```python
from build123d import *

# Parameters (mm, degrees)
SKETCH1_W           = 44.4
SKETCH1_H           = 40
SKETCH1_R           = 2.6
BOSS_EXTRUDE1_DEPTH = 2
SKETCH2_W           = 44.4
SKETCH2_H           = 18.3
BOSS_EXTRUDE2_DEPTH = 2
LPATTERN1_COUNT     = 2
LPATTERN1_PITCH     = 16.3
SKETCH3_R           = 2.6
CUT_EXTRUDE1_DEPTH  = 64.253853638
BOSS_EXTRUDE3_START = -22.2
SKETCH6_W           = 11.69
SKETCH6_H           = 16
BOSS_EXTRUDE3_DEPTH = 44.4
FILLET4_SIZE        = 1
SKETCH11_W          = 10
SKETCH11_H          = 5
CUT_EXTRUDE6_DEPTH  = 14
SKETCH12_W          = 10
SKETCH12_H          = 8.384441544
CUT_EXTRUDE7_DEPTH  = 11
SKETCH7_R           = 2.6
CUT_EXTRUDE2_DEPTH  = 9


with BuildPart() as part:
    # Sketch1 → Boss-Extrude1 (new body)
    with BuildSketch(Plane.XY):
        with Locations((22.2, 20)):
            Rectangle(SKETCH1_W, SKETCH1_H)
        with Locations((8, 8.476902454)):
            Circle(SKETCH1_R, mode=Mode.SUBTRACT)
        with Locations((8, 29.976902454)):
            Circle(SKETCH1_R, mode=Mode.SUBTRACT)
        with Locations((36.4, 29.976902454)):
            Circle(SKETCH1_R, mode=Mode.SUBTRACT)
        with Locations((36.4, 8.476902454)):
            Circle(SKETCH1_R, mode=Mode.SUBTRACT)
    boss_extrude1 = extrude(amount=BOSS_EXTRUDE1_DEPTH)

    # Sketch2 → Boss-Extrude2 (add)
    with BuildSketch(Plane(origin=(0, 40, 0), x_dir=(1, 0, 0), z_dir=(0, 1, 0))):
        with Locations((22.2, 7.15)):
            Rectangle(SKETCH2_W, SKETCH2_H)
    extrude(amount=BOSS_EXTRUDE2_DEPTH)

    # LPattern1: Boss-Extrude1 ×2
    with Locations(*[(0, 0, -i * LPATTERN1_PITCH) for i in range(1, LPATTERN1_COUNT)]):
        add(boss_extrude1)

    # Sketch3 → Cut-Extrude1 (cut, through all)
    with BuildSketch(Plane(origin=(0, 42, 0), x_dir=(1, 0, 0), z_dir=(0, 1, 0))):
        with Locations(Location((12.2, 7.15, 0), (0, 0, 270))):
            Circle(SKETCH3_R)
        with Locations(Location((32.2, 7.15, 0), (0, 0, 270))):
            Circle(SKETCH3_R)
    extrude(amount=-CUT_EXTRUDE1_DEPTH, mode=Mode.SUBTRACT)

    # Sketch6 → Boss-Extrude3 (add)
    with BuildSketch(Plane(origin=(22.2, 0, 0), x_dir=(0, 0, -1), z_dir=(1, 0, 0)).offset(BOSS_EXTRUDE3_START)):
        with Locations((-7.845, 34)):
            Rectangle(SKETCH6_W, SKETCH6_H)
    extrude(amount=BOSS_EXTRUDE3_DEPTH)

    # Fillet4
    fillet4_edges = [part.edges().sort_by_distance(p)[0] for p in [
        (44.4, 13, 2),
        (0, 21, -16.3),
        (44.4, 21, -16.3),
        (0, 42, -1.305),
        (44.4, 42, -1.305),
        (22.2, 42, -16.3),
        (22.2, 40, -14.3),
        (22.2, 0, -16.3),
        (0, 0, -15.3),
        (44.4, 0, -15.3),
        (22.2, 40, 0),
        (0, 13, 2),
        (44.4, 26, 7.845),
        (44.4, 34, 13.69),
        (22.2, 42, 13.69),
        (0, 26, 7.845),
        (0, 34, 13.69),
        (44.4, 0, 1),
        (0, 0, 1),
        (22.2, 0, 2),
    ]]
    chamfer(fillet4_edges, length=FILLET4_SIZE)

    # Sketch11 → Cut-Extrude6 (cut)
    with BuildSketch(Plane(origin=(0, 42, 0), x_dir=(1, 0, 0), z_dir=(0, 1, 0))):
        with Locations((22.2, -7.19)):
            Rectangle(SKETCH11_W, SKETCH11_H)
    extrude(amount=-CUT_EXTRUDE6_DEPTH, mode=Mode.SUBTRACT)

    # Sketch12 → Cut-Extrude7 (cut)
    with BuildSketch(Plane.XZ.offset(-26)):
        with Locations((8, 6.192220772)):
            Rectangle(SKETCH12_W, SKETCH12_H)
        with Locations((36.4, 6.192220772)):
            Rectangle(SKETCH12_W, SKETCH12_H)
    extrude(amount=-CUT_EXTRUDE7_DEPTH, mode=Mode.SUBTRACT)

    # Sketch7 → Cut-Extrude2 (cut)
    with BuildSketch(Plane.XY.offset(13.69)):
        with Locations((22.2, 32.73)):
            Circle(SKETCH7_R)
    extrude(amount=-CUT_EXTRUDE2_DEPTH, mode=Mode.SUBTRACT)


solid = part.part
```
The listing builds one solid part. Answer for the finished solid, in the listing's coordinates (mm). A direction names the side the tool comes from. Give positions to 0.01 mm unless a question says otherwise; leave off trailing zeros. Order: outer loops, then holes, each group sorted by start corner. A loop starts at its lowest first (then second) coordinate and runs counter-clockwise, first axis right, second up. Notation, with made-up numbers: M -3.5,69.25 L 53.5,69.25 A10 cw 53.5,73.25 Z; hole C -10,-27.75 d8. An arc over 180 degrees is marked long. Put each result on its own line as item: value. Start each with the question number.
Item 1: The part is cut by section C-C, the plane z = 11. Determine the outline of the cut face in (x, y), and give its area (3 significant figures).
Item 2: The part is cut by section B-B, the plane y = 23. Determine the outline of the cut face in (x, z), and give its area (3 significant figures).
Item 3: For a pull along Y with two mould halves and no side action, classify faces 5 (the face through (13, 31, 6)), 6 (the face through (10.4, 28.98, -15.31)), 7 (the face through (22, 42, -1)) as +Y half, -Y half, draft (parallel to the pull), parting line (faces both ways), or undercut.
Item 4: Flat-ended cylindrical pins translate along their axes: P1, Ø4.5, axis at x = 36.4, y = 8.48, coming from the +Z side; P2, Ø4, axis at x = 9, z = 5, coming from the -Y side; P3, Ø3.5, axis at x = 23, z = -10, coming from the -Y side; P4, Ø1.5, axis at x = 5.5, y = 20, coming from the +Z side. Find the tip coordinate at first contact, or state that the pin passes through.
Item 5: Which of the six approach directions +Z, -Z, +X, -X, +Y, -Y give full straight-line access (tool end or side, diameter ignored) to faces 1 (the face through (34.34, 28.39, 0.99)), 2 (the face through (27.2, 35, 7)), 3 (the face through (22, 15, 2)), 4 (the face through (22, 26, 9))?
Item 6: Find the intervals of material crossed by line 1 along Z through (x, y) = (12, 29.5); line 2 along Z through (x, y) = (17, 10.5); line 3 along Y through (x, z) = (8, -15.7), in increasing order.
Item 7: The part is cut by section A-A, the plane x = 22.2. Determine the outline of the cut face in (y, z), and give its area (3 significant figures).
Item 8: The part is cut by section D-D, the plane x = 36.4. State how many separate pieces and enclosed holes the cut face has, and give its area (3 significant figures).
Answer key:
1. outline: M 0,27 L 1,26 L 43.4,26 L 44.4,27 L 44.4,41 L 43.4,42 L 1,42 L 0,41 Z; hole C 22.2,32.73 d5.2
1. area: 687 mm²
2. outline: M 0,-15.3 L 1,-16.3 L 43.4,-16.3 L 44.4,-15.3 L 44.4,-14.3 L 0,-14.3 Z; M 0,0 L 44.4,0 L 44.4,1 L 43.4,2 L 1,2 L 0,1 Z
2. area: 176 mm²
3. face 5: draft
3. face 6: undercut
3. face 7: +Y half
4. P1: passes through
4. P2: stops at y = 37
4. P3: stops at y = 40
4. P4: stops at z = 2
5. face 1: -Z
5. face 2: +Y
5. face 3: -Y
5. face 4: +Z, +X, -X, -Y
6. line 1: z = -16.3 to -14.3, 0 to 2, 10.38 to 13.69
6. line 2: z = -16.3 to -14.3, 0 to 2
6. line 3: y = 0.4 to 5.88, 11.08 to 27.38, 32.58 to 41.6
7. outline: M 0,-15.3 L 1,-16.3 L 41,-16.3 L 42,-15.3 L 42,4.69 L 28,4.69 L 28,9.69 L 30.13,9.69 L 30.13,13.69 L 26,13.69 L 26,2 L 1,2 L 0,1 L 0,0 L 39,0 L 40,-1 L 40,-13.3 L 39,-14.3 L 0,-14.3 Z; M 35.33,9.69 L 42,9.69 L 42,12.69 L 41,13.69 L 35.33,13.69 Z
7. area: 292 mm²
8. separate pieces: 5
8. enclosed holes: 0
8. area: 249 mm²
